Geometry check sheet. Reference: drawing and pictorial views, mm from the part's lowest x, y, z. Give positions to 0.01 mm unless a question says otherwise; leave off trailing zeros. Write each loop counter-clockwise with the first axis right and the second up, starting at its lowest first coordinate (ties: lowest second). Pieces come first, ordered by that corner, then holes. Notation, with made-up numbers: M -25.75,-9.5 L -7.75,-9.5 A21 ccw -7.75,25.5 Z; hole C -33.5,87 d8. An arc over 180 degrees is marked long. Answer as a JSON object with one key per item and string values.
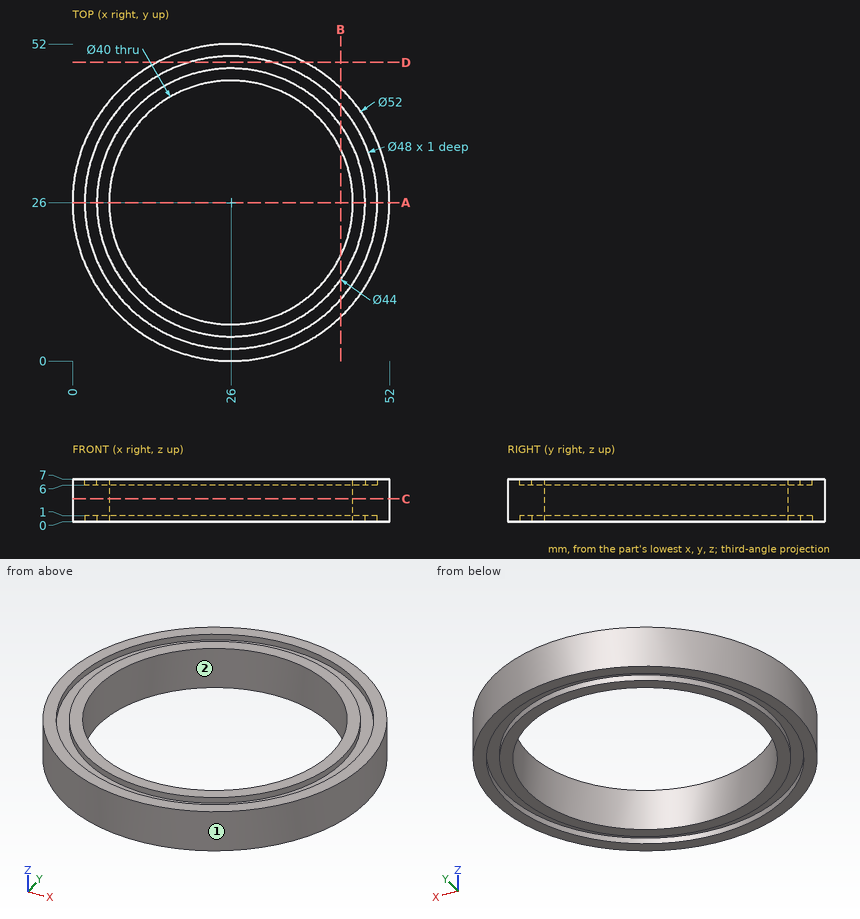
1) Thickness scan on L1, parallel to Y at x = 26, z = 0.6; L2, parallel to Y at x = 8, z = 6.25; L3, parallel to X at y = 23.5, z = 6.75. Record the ranges inside material, lowest first.
Completed:
{"L1": "y = 0 to 2, 4 to 6, 46 to 48, 50 to 52", "L2": "y = 7.24 to 10.13, 13.35 to 17.28, 34.72 to 38.65, 41.87 to 44.76", "L3": "x = 0.12 to 2.13, 4.14 to 6.16, 45.84 to 47.86, 49.87 to 51.88"}
2) Section check D-D on y = 49. Record the boundary of the cut face in (x, z).
Completed:
{"outline": "M 13.88,0 L 19.14,0 L 19.14,1 L 32.86,1 L 32.86,0 L 38.12,0 L 38.12,7 L 32.86,7 L 32.86,6 L 19.14,6 L 19.14,7 L 13.88,7 Z"}
3) Section check A-A on y = 26. Record the boundary of the cut face in (x, z).
Completed:
{"outline": "M 0,0 L 2,0 L 2,1 L 4,1 L 4,0 L 6,0 L 6,7 L 4,7 L 4,6 L 2,6 L 2,7 L 0,7 Z; M 46,0 L 48,0 L 48,1 L 50,1 L 50,0 L 52,0 L 52,7 L 50,7 L 50,6 L 48,6 L 48,7 L 46,7 Z"}
4) Section check B-B on x = 44. Record the boundary of the cut face in (y, z), and give its area (3 significant figures).
Completed:
{"outline": "M 7.24,0 L 10.13,0 L 10.13,1 L 13.35,1 L 13.35,0 L 17.28,0 L 17.28,7 L 13.35,7 L 13.35,6 L 10.13,6 L 10.13,7 L 7.24,7 Z; M 34.72,0 L 38.65,0 L 38.65,1 L 41.87,1 L 41.87,0 L 44.76,0 L 44.76,7 L 41.87,7 L 41.87,6 L 38.65,6 L 38.65,7 L 34.72,7 Z", "area": "128 mm2"}
5) Release check for a two-part mould opening along Y. For the marked faces 1 and 2 record: pulls with the +Y half, pulls with the -Y half, needs draft (parallel to the pull), parting line crosses it, or undercut.
Completed:
{"face 1": "parting line crosses it", "face 2": "undercut"}
6) Go/stop test with flat-tipped pins: pin 1 (10 mm diameter, centred on x = 29.5, y = 37, fed in from +Z); pin 2 (4 mm diameter, centred on y = 46, z = 3.5, fed in from -X). Record where each tip stops, or that it passes through.
Completed:
{"pin 1": "passes through", "pin 2": "stops at x = 7.24"}
7) Section check C-C on z = 3.75. Record the boundary of the cut face in (x, y).
Completed:
{"outline": "C 26,26 d52; hole C 26,26 d40"}
